Geometry check sheet. Reference: the model listing, model coordinates, mm. Round coordinates to 2 decimals unless told otherwise and drop trailing zeros. Order: outer loops, then holes, each group sorted by start corner. A loop starts at its lowest first (then second) coordinate and runs counter-clockwise, first axis right, second up. Notation, with made-up numbers: (63.25, 81.5) - (87.25, 81.5) arc R16 cw to (87.25, 104.5) - close; hole circle Ø6 at (48.5, 18.5). An arc over 180 degrees is marked (long way). Return JSON: item names as keys, results as strings. Group by question number.
Q1. Sectioned sample at A-A, the plane y = -1.6. Record the cut outline in (x, z), then the cut area to 3 significant figures.
Q2. Sectioned sample at C-C, the plane x = 28. Record the cut outline in (y, z), then the cut area to 3 significant figures.
Q3. Gauge pin test, flat ends, axial feed: pin 1 Ø1 at (x, y) = (-18, -2) entering from +Z; pin 2 Ø0.6 at (x, y) = (-24.5, -1) entering from +Z. Record the tip position at first contact, or that the pin passes through.
Q4. Sectioned sample at B-B, the plane x = -3. Record the cut outline in (y, z), then the cut area to 3 significant figures.
Q5. Material ranges on line 1 along X through (y, z) = (-0.35, -4.5); line 2 along Z through (x, y) = (-1, -1.4); line 3 along Z through (x, y) = (-28, -0.4), recorded low to high.
```python
from build123d import *

# Parameters (mm, degrees)
F1_DEPTH = 2


with BuildPart() as f1:
    # F0 (on Front) → F1 (new body)
    with BuildSketch(Plane.XZ):
        with BuildLine():
            Line((-30, 5), (-35, 5))
            Line((-35, 5), (-35, 1.5))
            Line((-35, 1.5), (-35, -1.5))
            Line((-35, -1.5), (-35, -5))
            Line((-35, -5), (-30, -5))
            Line((-30, -5), (-30, -3))
            Line((-30, -3), (-20.267827, -3))
            ThreePointArc((-20.267827, -3), (-17.738613, -1.882308), (-15, -1.5))
            Line((-15, -1.5), (15, -1.5))
            ThreePointArc((15, -1.5), (17.738613, -1.882308), (20.267827, -3))
            Line((20.267827, -3), (30, -3))
            Line((30, -3), (30, -5))
            Line((30, -5), (35, -5))
            Line((35, -5), (35, -1.5))
            Line((35, -1.5), (35, 1.5))
            Line((35, 1.5), (35, 5))
            Line((35, 5), (30, 5))
            Line((30, 5), (30, 3))
            Line((30, 3), (20.267827, 3))
            ThreePointArc((20.267827, 3), (17.738613, 1.882308), (15, 1.5))
            Line((15, 1.5), (-15, 1.5))
            ThreePointArc((-15, 1.5), (-17.738613, 1.882308), (-20.267827, 3))
            Line((-20.267827, 3), (-30, 3))
            Line((-30, 3), (-30, 5))
        make_face()
    extrude(amount=F1_DEPTH)


solid = f1.part
```
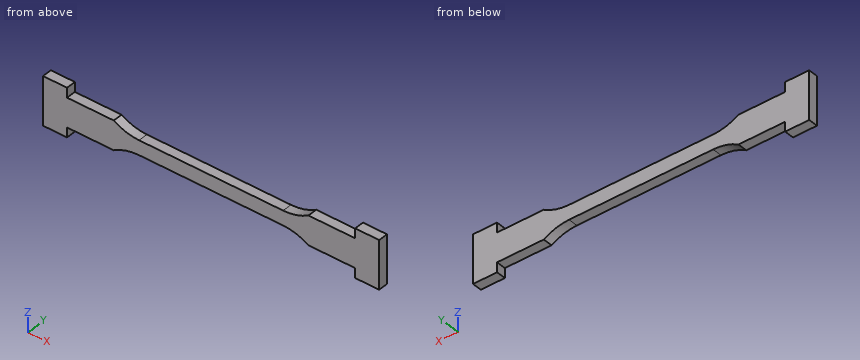
Reply:
{
 "1": {"outline": "(-35, -5) - (-30, -5) - (-30, -3) - (-20.27, -3) arc R10 cw to (-15, -1.5) - (15, -1.5) arc R10 cw to (20.27, -3) - (30, -3) - (30, -5) - (35, -5) - (35, 5) - (30, 5) - (30, 3) - (20.27, 3) arc R10 cw to (15, 1.5) - (-15, 1.5) arc R10 cw to (-20.27, 3) - (-30, 3) - (-30, 5) - (-35, 5) - close", "area": "349 mm^2"},
 "2": {"outline": "(-2, -3) - (0, -3) - (0, 3) - (-2, 3) - close", "area": "12.0 mm^2"},
 "3": {"pin 1": "z = 2.13", "pin 2": "z = 3"},
 "4": {"outline": "(-2, -1.5) - (0, -1.5) - (0, 1.5) - (-2, 1.5) - close", "area": "6.00 mm^2"},
 "5": {"line 1": "-35 to -30, 30 to 35", "line 2": "-1.5 to 1.5", "line 3": "-3 to 3"}
}
